Input: part model. Units: mm. Frame: model coordinates. Give positions to 0.01 mm unless a question says otherwise; leave off trailing zeros. Write each loop counter-clockwise with the first axis right and the second up, starting at its lowest first coordinate (ties: lowest second). Pieces come first, ordered by that corner, then holes. Notation, with made-up numbers: (37.5, -28.5) -> (76.5, -28.5) arc R25 ccw to (76.5, 0.5) -> close; hole circle Ø1 at (76.25, 47.25). An arc over 180 degrees is marked (long way). Return JSON: item names as keys, results as strings. Group by question number.
Item 1: Section A-A, the plane z = -3.05. Return loops of the section in (x, y), then the cut area to 3 significant figures.
Item 2: Section D-D, the plane y = 53. Return loops of the section in (x, z), then the cut area to 3 significant figures.
Item 3: Pin query (flat end, axial travel): P1, Ø1.5, axis at x = 2.5, z = -2.5, coming from the -Y side; P2, Ø0.9, axis at x = -6, z = -3, coming from the -Y side. Return the tip coordinate at first contact, or that it passes through.
Item 4: Line query: line 1 (X direction, y = 35, z = -3.55); line 2 (Y direction, x = -31, z = -3.45); line 3 (Y direction, x = -0.5, z = -3.5). Output: solid intervals per line, ascending. Write a range as [from, to].
Item 5: Section B-B, the plane x = 12. Return loops of the section in (y, z), then the cut area to 3 significant figures.
Item 6: Section C-C, the plane y = 15. Return loops of the section in (x, z).
Solid Edge part; units mm, degrees
sketch "Sketch1" plane through (0, 0, 0) normal (0, 0, 1) x (1, 0, 0)
  line L0 (-35, -40) -> (35, -40)
  line L1 (35, -40) -> (35, 40)
  line L2 (35, 40) -> (-35, 40)
  line L3 (-35, 40) -> (-35, -40)
extrude "Protrusion1" add sketch "Sketch1" along normal blind 25
sketch "Sketch2" plane through (0, -40, 12.5) normal (0, -1, 0) x (1, 0, 0)
  line L0 (-24, 8.5) -> (-24, 2.5)
  line L1 (-24, 2.5) -> (0, 2.5)
  line L2 (24, 2.5) -> (0, 2.5)
  line L3 (24, 8.5) -> (24, 2.5)
  line L4 (20, 8.5) -> (24, 8.5)
  line L5 (20, 12.5) -> (20, 8.5)
  line L6 (20, 12.5) -> (0, 12.5)
  line L7 (-20, 12.5) -> (0, 12.5)
  line L8 (-20, 12.5) -> (-20, 8.5)
  line L9 (-20, 8.5) -> (-24, 8.5)
extrude "ExtrudedCutout_1" cut sketch "Sketch2" against normal blind 70
sketch "Sketch3" plane through (35, 0, 12.5) normal (1, 0, 0) x (0, 1, 0)
  line L0 (-17, 12.5) -> (-40, 12.5)
  line L1 (-40, 12.5) -> (-40, 2.5)
  line L2 (-40, 2.5) -> (-29, 2.5)
  line L3 (-29, 2.5) -> (-17, 12.5)
extrude "ExtrudedCutout_2" cut sketch "Sketch3" against normal blind 153.7771
sketch "Sketch4" plane through (0, -5, 15) normal (0, 0, 1) x (1, 0, 0)
  line L0 (-35, -24) -> (-35, -35)
  line L1 (-35, -35) -> (-16, -35)
  line L2 (-21, -24) -> (-16, -35)
  line L3 (-35, -24) -> (-21, -24)
  line L4 (21, -24) -> (16, -35)
  line L5 (35, -35) -> (16, -35)
  line L6 (35, -24) -> (35, -35)
  line L7 (21, -24) -> (35, -24)
extrude "ExtrudedCutout_3" cut sketch "Sketch4" against normal blind 32.0943
fillet "Round_1" radius 4 10 edges at (-35, -29, 7.5) (-28, -29, 0) (35, -29, 7.5) (28, -29, 0) (-18.5, -34.5, 0) (18.5, -34.5, 0) (0, -40, 0) (0, -40, 15) (-18.5, -34.5, 15) (18.5, -34.5, 15)
sketch "Sketch5" plane through (0, -3, 15) normal (0, 0, 1) x (1, 0, 0)
  line L0 (0, 22) -> (-14.5, 22)
  line L1 (-14.5, 36.4868) -> (-14.5, 22)
  line L2 (-14.5, 36.4868) -> (14.5, 36.4868)
  line L3 (14.5, 36.4868) -> (14.5, 22)
  line L4 (0, 22) -> (14.5, 22)
extrude "ExtrudedProtrusion_2" add sketch "Sketch5" along normal blind 10
sketch "Sketch6" plane through (0, 19, 20) normal (0, -1, 0) x (1, 0, 0)
  line L0 (-4.5, 4) -> (-4.5, -5)
  line L1 (-4.5, -5) -> (-3.5, -5)
  line L2 (-3.5, -5) -> (-3.5, 4)
  line L3 (-3.5, 4) -> (-4.5, 4)
  line L4 (-12.5, 4) -> (-12.5, -5)
  line L5 (-11.5, -5) -> (-12.5, -5)
  line L6 (-11.5, 4) -> (-11.5, -5)
  line L7 (-12.5, 4) -> (-11.5, 4)
  line L8 (11.5, 4) -> (11.5, -5)
  line L9 (11.5, -5) -> (12.5, -5)
  line L10 (12.5, -5) -> (12.5, 4)
  line L11 (12.5, 4) -> (11.5, 4)
extrude "Cutout1" cut sketch "Sketch6" against normal up to vertex (11 mm away)
sketch "Sketch7" plane through (0, 2, 0) normal (0, 0, -1) x (1, 0, 0)
  line L0 (14.5, -28) -> (-14.5, -28)
  line L1 (-14.5, -28) -> (-14.5, -21.6722)
  line L2 (-14.5, -21.6722) -> (14.5, -21.6722)
  line L3 (14.5, -21.6722) -> (14.5, -28)
extrude "ExtrudedCutout_6" cut sketch "Sketch7" against normal blind 20
sketch "Sketch8" plane through (0, 2, 0) normal (0, 0, -1) x (1, 0, 0)
  line L0 (-6.5737, 62.269) -> (-33.7882, 46.8229)
  arc A0 (-33.7882, 46.8229) -> (-37, 41.3069) centre (-30.6575, 41.3069) ccw
  line L1 (-37, 41.3069) -> (-37, 2)
  line L2 (-37, -37.3069) -> (-37, 2)
  arc A1 (-33.7882, -42.8229) -> (-37, -37.3069) centre (-30.6575, -37.3069) cw
  line L3 (-6.5737, -58.269) -> (-33.7882, -42.8229)
  arc A2 (-6.5737, -58.269) -> (0, -60.0045) centre (0, -46.6867) ccw
  arc A3 (6.5737, -58.269) -> (0, -60.0045) centre (0, -46.6867) cw
  line L4 (6.5737, -58.269) -> (33.7882, -42.8229)
  arc A4 (33.7882, -42.8229) -> (37, -37.3069) centre (30.6575, -37.3069) ccw
  line L5 (37, -37.3069) -> (37, 2)
  line L6 (37, 41.3069) -> (37, 2)
  arc A5 (33.7882, 46.8229) -> (37, 41.3069) centre (30.6575, 41.3069) cw
  line L7 (6.5737, 62.269) -> (33.7882, 46.8229)
  arc A6 (6.5737, 62.269) -> (0, 64.0045) centre (0, 50.6867) ccw
  arc A7 (-6.5737, 62.269) -> (0, 64.0045) centre (0, 50.6867) cw
extrude "ExtrudedProtrusion_3" add sketch "Sketch8" along normal blind 5
sketch "Sketch9" plane through (0, -3, 15) normal (0, 0, 1) x (0, -1, 0)
  line L0 (33, 13) -> (25, 13)
  line L1 (25, 13) -> (25, -13)
  line L2 (25, -13) -> (33, -13)
  line L3 (33, -13) -> (33, 0)
  line L4 (33, 0) -> (33, 13)
extrude "Cutout2" cut sketch "Sketch9" against normal blind 5
fillet "Round_2" radius 4 3 edges at (35, 40, 12.5) (0, 40, 25) (-35, 40, 12.5)
fillet "Round_3" radius 2 12 edges at (-20.181, -52.5459, 0) (-36.1385, -42.4984, 0) (-37, 0, 0) (-36.1385, 42.4984, 0) (-20.181, 52.5459, 0) (0, 62.0045, 0) (20.181, 52.5459, 0) (36.1385, 42.4984, 0) (37, 0, 0) (36.1385, -42.4984, 0) (20.181, -52.5459, 0) (0, -62.0045, 0)
sketch "Sketch10" plane through (0, 0, -5) normal (0, 0, -1) x (0, -1, 0)
  circle A0 centre (-26.0045, 31) radius 1.0001
  circle A1 centre (26.0045, 31) radius 1.0001
  circle A2 centre (-26.0045, -31) radius 1.0001
  circle A3 centre (26.0045, -31) radius 1.0001
extrude "ExtrudedCutout_9" cut sketch "Sketch10" against normal blind 10
sketch "Sketch11" plane through (-35, 5.5, 12.5) normal (-1, 0, 0) x (0, -1, 0)
  line L0 (-60.0023, -4.5) -> (-60.0023, -14.5)
  line L1 (-60.0023, -14.5) -> (90.1927, -14.5)
  line L2 (90.1927, -4.5) -> (90.1927, -14.5)
  line L3 (90.1927, 27.3922) -> (90.1927, -4.5)
  line L4 (-13.5, 27.3922) -> (90.1927, 27.3922)
  line L5 (-13.5, 27.3922) -> (-60.0023, 27.3922)
  line L6 (-60.0023, 27.3922) -> (-60.0023, -4.5)
extrude "Cutout3" cut sketch "Sketch11" along normal mid plane 351.619
sketch "Sketch12" plane through (0, 0, -5) normal (0, 0, -1) x (0, -1, 0)
  line L0 (-38.9803, 21.8154) -> (-8.3641, 21.8173)
  line L1 (-8.3641, 21.8173) -> (-8.3641, -19.6643)
  line L2 (-8.3641, -19.6643) -> (-38.9803, -19.6643)
  line L3 (-38.9803, -19.6643) -> (-38.9803, 21.8154)
extrude "ExtrudedCutout_13" cut sketch "Sketch12" along normal mid plane 51.4806
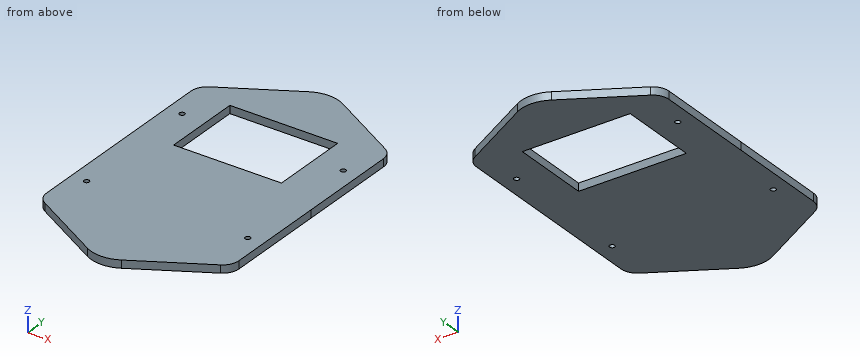
Answer below:
{
 "1": {"outline": "(-37, -39.31) arc R6.34 ccw to (-33.79, -44.82) -> (-6.57, -60.27) arc R13.32 ccw to (6.57, -60.27) -> (33.79, -44.82) arc R6.34 ccw to (37, -39.31) -> (37, 0) -> (37, 39.31) arc R6.34 ccw to (33.79, 44.82) -> (6.57, 60.27) arc R13.32 ccw to (-6.57, 60.27) -> (-33.79, 44.82) arc R6.34 ccw to (-37, 39.31) -> (-37, 0) -> close; hole circle Ø2 at (-31, -26); hole circle Ø2 at (-31, 26); hole (-21.82, 8.36) -> (19.66, 8.36) -> (19.66, 38.98) -> (-21.82, 38.98) -> close; hole circle Ø2 at (31, -26); hole circle Ø2 at (31, 26)", "area": "6,610 mm2"},
 "2": {"outline": "(-19.38, -5) -> (19.38, -5) -> (19.38, -2) -> (-19.38, -2) -> close", "area": "116 mm2"},
 "3": {"P1": "stops at y = -61.89", "P2": "stops at y = -60.79"},
 "4": {"line 1": "x = [-37, -21.82], [19.66, 37]", "line 2": "y = [-46.41, -27], [-25, 25], [27, 46.41]", "line 3": "y = [-62, 8.36], [38.98, 62]"},
 "5": {"outline": "(-57.19, -5) -> (8.36, -5) -> (8.36, -2) -> (-57.19, -2) -> close; (38.98, -5) -> (57.19, -5) -> (57.19, -2) -> (38.98, -2) -> close", "area": "251 mm2"},
 "6": {"outline": "(-37, -5) -> (-21.82, -5) -> (-21.82, -2) -> (-37, -2) -> close; (19.66, -5) -> (37, -5) -> (37, -2) -> (19.66, -2) -> close"}
}
